Can you work these out from the drawing? Everything is in mm from the part's minimum corner. A direction names the side the tool comes from. Coordinates: 2 decimals unless noted, no trailing zeros. Order: outer loops, then holes, each group sorted by start corner. A loop starts at its lowest first (then second) coordinate and runs counter-clockwise, first axis right, second up. Notation, with made-up numbers: (6, 51) -> (11, 51) arc R20 cw to (11, 77) -> close; hole circle Ø7 at (83, 65). An arc over 180 degrees is marked (long way). Answer in a Markdown table with one row per item.
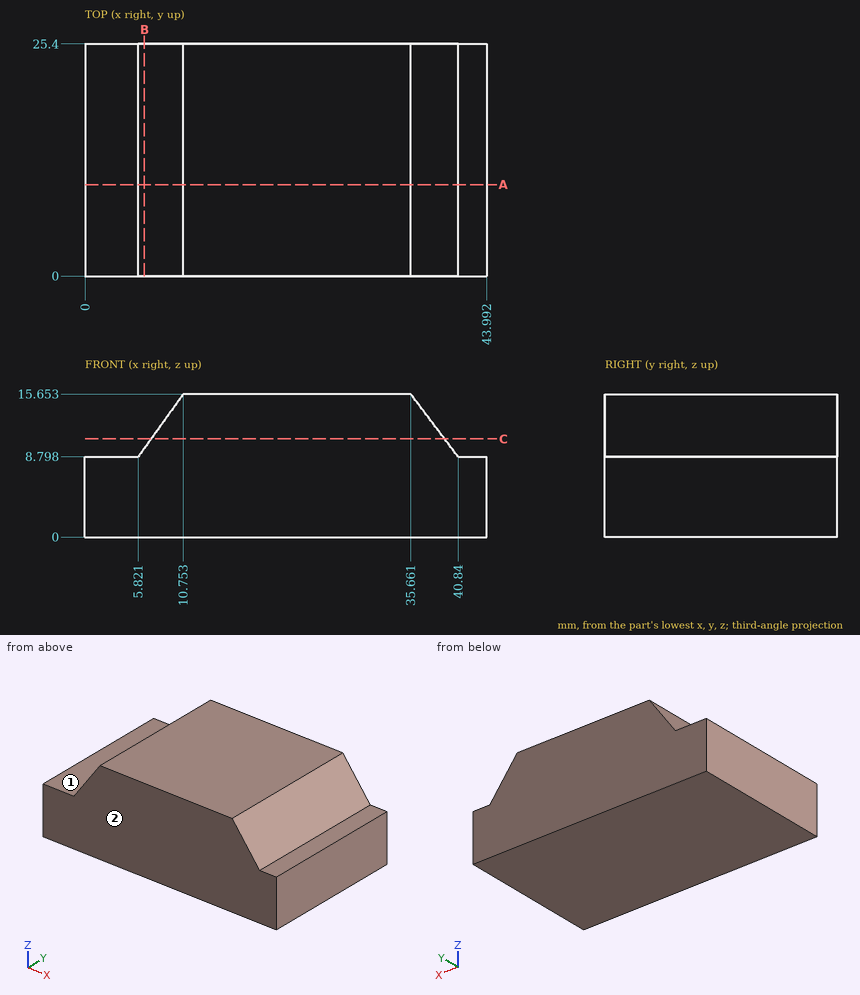
(1) I need wall thicknesses on line 1 (Z direction, x = 3.5, y = 2.25); line 2 (X direction, y = 24.5, z = 12.25) (1 decimal); line 3 (X direction, y = 10.75, z = 10.25) (1 decimal). Which ranges of each line are inside material? Lowest first, please. Write a range as [from, to].
Response values:
| item | result |
|---|---|
| line 1 | [0, 8.8] |
| line 2 | [8.3, 38.2] |
| line 3 | [6.9, 39.7] |
(2) On a 3-axis mill with a long thin cutter (end or side, diameter ignored), from which of +Z, -Z, +X, -X, +Y, -Y can I reach the whole of each face in a straight line? I mean the marked faces 1 and 2. Say none if no direction works.
Response values:
| item | result |
|---|---|
| face 1 | +Z, -X, +Y, -Y |
| face 2 | +Z, -Z, +X, -X, -Y |
(3) Suppose I cut it at B-B (x = 6.5). Please give me the cut outline in (y, z).
Response values:
| item | result |
|---|---|
| outline | (0, 0) -> (25.4, 0) -> (25.4, 9.74) -> (0, 9.74) -> close |
(4) Suppose I cut it at A-A (y = 10). Please give me the cut outline in (x, z).
Response values:
| item | result |
|---|---|
| outline | (0, 0) -> (43.99, 0) -> (43.99, 8.8) -> (40.84, 8.8) -> (35.66, 15.65) -> (10.75, 15.65) -> (5.82, 8.8) -> (0, 8.8) -> close |
(5) Will these pins go through, and if not, where does the flat tip stop? pin 1 Ø6 at (x, z) = (27.5, 6) entering from -Y; pin 2 Ø3 at (x, y) = (3.5, 19) entering from +Z.
Response values:
| item | result |
|---|---|
| pin 1 | y = 0 |
| pin 2 | z = 8.8 |
(6) Suppose I cut it at C-C (z = 10.75). Please give me the cut outline in (x, y) (1 decimal), and give its area (3 significant figures).
Response values:
| item | result |
|---|---|
| outline | (7.2, 0) -> (39.4, 0) -> (39.4, 25.4) -> (7.2, 25.4) -> close |
| area | 816 mm2 |
